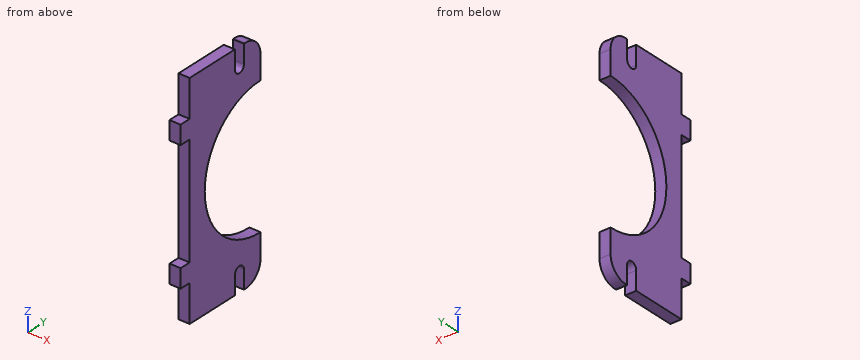
from build123d import *

# Parameters (mm, degrees)
BOSS_EXTRUDE1_DEPTH = 3
CUT_EXTRUDE2_DEPTH  = 4
FILLET2_R           = 5
SKETCH3_W           = 3
SKETCH3_H           = 5
BOSS_EXTRUDE2_DEPTH = 3


with BuildPart() as part:
    # Sketch1 → Boss-Extrude1 (new body)
    with BuildSketch(Plane(origin=(0, 0, 0), x_dir=(0, 0, -1), z_dir=(1, 0, 0))):
        with BuildLine():
            Line((-18.5, 11.75), (-30, 11.75))
            Line((-30, 11.75), (-30, -11.75))
            Line((-30, -11.75), (30, -11.75))
            Line((30, -11.75), (30, 11.75))
            Line((30, 11.75), (18.5, 11.75))
            ThreePointArc((18.5, 11.75), (0, -6.75), (-18.5, 11.75))
        make_face()
    extrude(amount=BOSS_EXTRUDE1_DEPTH)

    # Sketch2 → Cut-Extrude2 (cut, through all)
    with BuildSketch(Plane(origin=(3, 0, 0), x_dir=(0, 0, -1), z_dir=(1, 0, 0))):
        with BuildLine():
            Line((-25, 6.25), (-30, 6.25))
            Line((-30, 6.25), (-30, 3.25))
            Line((-30, 3.25), (-25, 3.25))
            ThreePointArc((-25, 3.25), (-23.5, 4.75), (-25, 6.25))
        make_face()
    cut_extrude2 = extrude(amount=-CUT_EXTRUDE2_DEPTH, mode=Mode.SUBTRACT)

    # Mirror2: Cut-Extrude2 across plane
    add(cut_extrude2.mirror(Plane.XY), mode=Mode.SUBTRACT)

    # Fillet2
    fillet2_edges = [part.edges().sort_by_distance(p)[0] for p in [
        (1.5, 11.75, 30),
        (1.5, 11.75, -30),
    ]]
    fillet(fillet2_edges, radius=FILLET2_R)

    # Sketch3 → Boss-Extrude2 (add)
    with BuildSketch(Plane.XZ.offset(11.75)):
        with Locations((1.5, -17.5)):
            Rectangle(SKETCH3_W, SKETCH3_H)
    boss_extrude2 = extrude(amount=BOSS_EXTRUDE2_DEPTH)

    # Mirror3: Boss-Extrude2 across plane
    add(boss_extrude2.mirror(Plane.XY))


solid = part.part
The listing builds one solid part. Answer for the finished solid, in the listing's coordinates (mm). Give positions to 0.01 mm unless a question says otherwise; leave off trailing zeros. Loops run counter-clockwise (first coordinate to the right, second up) from the corner with the lowest first, then second, coordinate; pieces in that order, holes last.
Item 1: A cutting plane is placed at A-A (x = 2.05). Give the vertices of the cut face in (y, z).
Derived:
outline: (-14.75, -20) - (-11.75, -20) - (-11.75, -30) - (3.25, -30) - (3.25, -25) arc R1.5 cw to (6.25, -25) - (6.25, -30) - (6.75, -30) arc R5 ccw to (11.75, -25) - (11.75, -18.5) arc R18.5 cw to (11.75, 18.5) - (11.75, 25) arc R5 ccw to (6.75, 30) - (6.25, 30) - (6.25, 25) arc R1.5 cw to (3.25, 25) - (3.25, 30) - (-11.75, 30) - (-11.75, 20) - (-14.75, 20) - (-14.75, 15) - (-11.75, 15) - (-11.75, -15) - (-14.75, -15) - close
Item 2: Each of these flat-tipped pins is pushed along its axis until it touches: pin 1 Ø1.5 at (x, y) = (2, -13.5) entering from +Z; pin 2 Ø1.5 at (x, y) = (1, -13.5) entering from -Z; pin 3 Ø1.5 at (x, z) = (1.5, -28) entering from -Y; pin 4 Ø3 at (y, z) = (8, 16) entering from +X. Where does it stop, or does it pass through?
Derived:
pin 1: stops at z = 20
pin 2: stops at z = -20
pin 3: stops at y = -11.75
pin 4: passes through
Item 3: A cutting plane is placed at D-D (y = 0.25). Give the vertices of the cut face in (x, z), then the cut area to 3 significant figures.
Derived:
outline: (0, -30) - (3, -30) - (3, -14.49) - (0, -14.49) - close; (0, 14.49) - (3, 14.49) - (3, 30) - (0, 30) - close
area: 93.1 mm2
Item 4: Find the intervals of material crossed by line 1 along Z through (x, y) = (2, 3.5); line 2 along Z through (x, y) = (2.15, 0); line 3 along Y through (x, z) = (1.7, 24), in increasing order.
Derived:
line 1: z = -24.17 to -16.56, 16.56 to 24.17
line 2: z = -30 to -14.29, 14.29 to 30
line 3: y = -11.75 to 3.63, 5.87 to 11.75
Item 5: A cutting plane is placed at C-C (z = 21). Give the vertices of the cut face in (x, y).
Derived:
outline: (0, -11.75) - (3, -11.75) - (3, 11.75) - (0, 11.75) - close
Item 6: A cutting plane is placed at B-B (y = 4.75). Give the vertices of the cut face in (x, z).
Derived:
outline: (0, -23.5) - (3, -23.5) - (3, -17.12) - (0, -17.12) - close; (0, 17.12) - (3, 17.12) - (3, 23.5) - (0, 23.5) - close
